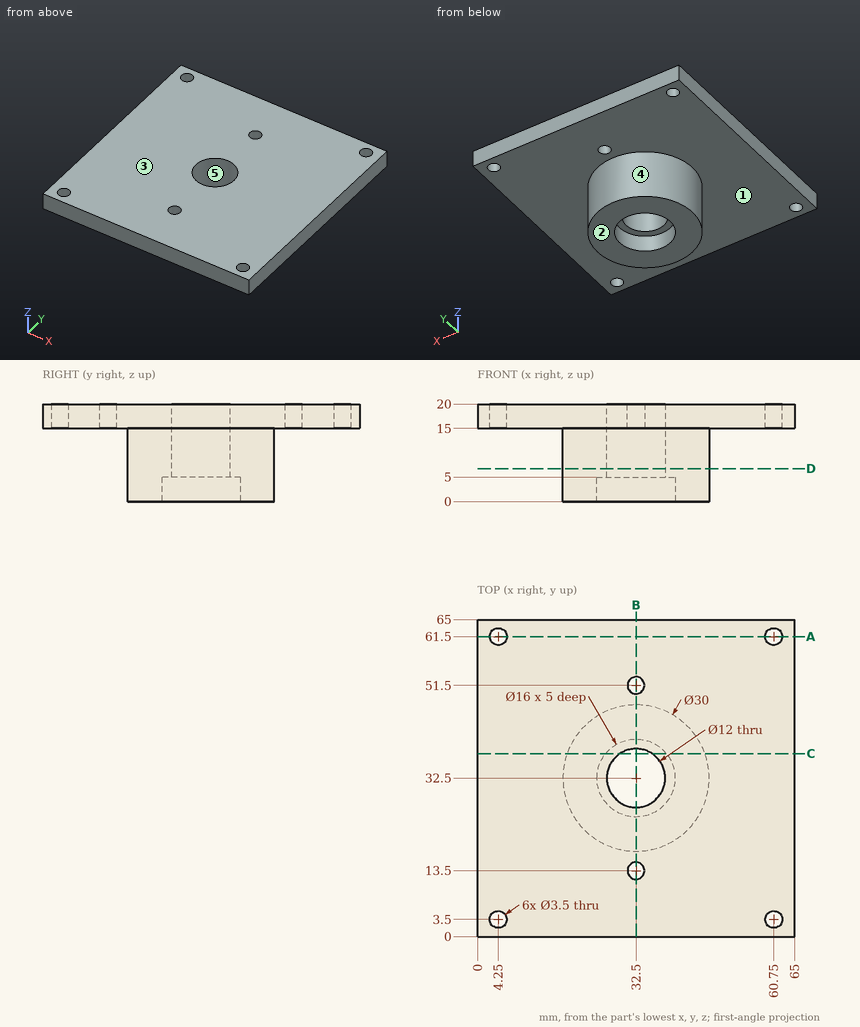
Here's the drawing with two shaded views (mm, measured from the low corner). I have some questions. A direction names the side the tool comes from. Give positions to 0.01 mm unless a question says otherwise; leave off trailing zeros. Order: outer loops, then holes, each group sorted by start corner. A loop starts at its lowest first (then second) coordinate and runs counter-clockwise, first axis right, second up. Notation, with made-up numbers: M 57,27 L 80,27 A28 cw 80,56 Z; hole C 8.5,38 d11. An arc over 180 degrees is marked long. One line per item, written item: value.
1) On a 3-axis mill with a long thin cutter (end or side, diameter ignored), from which of +Z, -Z, +X, -X, +Y, -Y can I reach the whole of each face in a straight line? I mean the marked faces 1 and 2. Say none if no direction works.
Answer sheet:
face 1: -Z
face 2: -Z, +X, -X, +Y, -Y
2) I want a section at A-A, the plane y = 61.5. List the corners of the cut face in (x, z) for me, plus the area to 3 significant figures.
Answer sheet:
outline: M 0,15 L 2.5,15 L 2.5,20 L 0,20 Z; M 6,15 L 59,15 L 59,20 L 6,20 Z; M 62.5,15 L 65,15 L 65,20 L 62.5,20 Z
area: 290 mm^2
3) For P1, Ø5.5, axis at x = 32.5, y = 13.5, coming from the -Z side; P2, Ø1, axis at y = 41.5, z = 3.5, coming from the -X side; P3, Ø12, axis at x = 50, z = 7, coming from the -Y side, each with a flat end and sliding along its axis, tell me the tip position at first contact or that it passes through.
Answer sheet:
P1: stops at z = 15
P2: stops at x = 20.14
P3: stops at y = 22.87
4) I want a section at B-B, the plane x = 32.5. List the corners of the cut face in (y, z) for me, plus the area to 3 significant figures.
Answer sheet:
outline: M 0,15 L 11.75,15 L 11.75,20 L 0,20 Z; M 15.25,15 L 17.5,15 L 17.5,0 L 24.5,0 L 24.5,5 L 26.5,5 L 26.5,20 L 15.25,20 Z; M 38.5,5 L 40.5,5 L 40.5,0 L 47.5,0 L 47.5,15 L 49.75,15 L 49.75,20 L 38.5,20 Z; M 53.25,15 L 65,15 L 65,20 L 53.25,20 Z
area: 480 mm^2
5) We'd pull the mould along X, two halves only. Please class the marked faces 3, 4 and 5: released by +X, released by -X, zero draft, split by the parting line, or undercut.
Answer sheet:
face 3: zero draft
face 4: split by the parting line
face 5: undercut
6) Please list where these lines run through material, in increasing order: line 1 along Y through (x, z) = (60.75, 16.25); line 2 along Y through (x, z) = (32.5, 16.9); line 3 along Y through (x, z) = (32.5, 4.05).
Answer sheet:
line 1: y = 0 to 1.75, 5.25 to 59.75, 63.25 to 65
line 2: y = 0 to 11.75, 15.25 to 26.5, 38.5 to 49.75, 53.25 to 65
line 3: y = 17.5 to 24.5, 40.5 to 47.5
7) I want a section at D-D, the plane z = 6.75. List the corners of the cut face in (x, y) for me, plus the area to 3 significant figures.
Answer sheet:
outline: C 32.5,32.5 d30; hole C 32.5,32.5 d12
area: 594 mm^2
8) I want a section at C-C, the plane y = 37.5. List the corners of the cut face in (x, z) for me (3 decimals).
Answer sheet:
outline: M 0,15 L 18.358,15 L 18.358,0 L 26.255,0 L 26.255,5 L 29.183,5 L 29.183,20 L 0,20 Z; M 35.817,5 L 38.745,5 L 38.745,0 L 46.642,0 L 46.642,15 L 65,15 L 65,20 L 35.817,20 Z
